```python
from build123d import *

# Parameters (mm, degrees)
BOSS_EXTRUDE2_DEPTH = 5
SKETCH3_W           = 9
SKETCH3_H           = 10
BOSS_EXTRUDE3_DEPTH = 4
SKETCH4_R           = 2.5
CUT_EXTRUDE1_DEPTH  = 10
FILLET1_R           = 1.75


with BuildPart() as part:
    # Sketch1 → Boss-Extrude2 (new body)
    with BuildSketch(Plane(origin=(0, 0, 0), x_dir=(1, 0, 0), z_dir=(0, 1, 0))):
        Polygon((0, 0), (-2, 9), (11, 9), (9, 0), (9, -10), (0, -10), align=None)
    extrude(amount=BOSS_EXTRUDE2_DEPTH)

    # Sketch3 → Boss-Extrude3 (add)
    with BuildSketch(Plane.XZ):
        with Locations((4.5, 5)):
            Rectangle(SKETCH3_W, SKETCH3_H)
    extrude(amount=BOSS_EXTRUDE3_DEPTH)

    # Sketch4 → Cut-Extrude1 (cut, through all)
    with BuildSketch(Plane.XZ.offset(4)):
        with Locations((4.5, 5)):
            Circle(SKETCH4_R)
    extrude(amount=-CUT_EXTRUDE1_DEPTH, mode=Mode.SUBTRACT)

    # Fillet1
    fillet1_edges = [part.edges().sort_by_distance(p)[0] for p in [
        (9, 5, 5),
        (10, 5, -4.5),
        (4.5, 5, -9),
        (-1, 5, -4.5),
        (0, 5, 5),
        (4.5, 5, 10),
    ]]
    fillet(fillet1_edges, radius=FILLET1_R)


solid = part.part
```
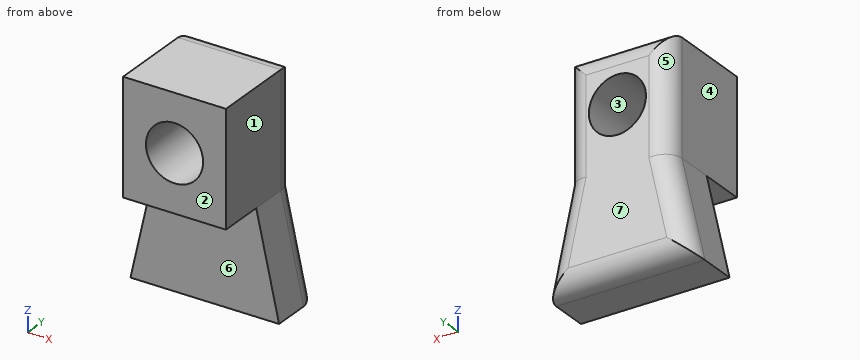
Could you check a few things on this model? Use its own coordinates, in mm. Face numbers are marked on the shaded views. A direction names the side the tool comes from. Coordinates: 2 decimals unless noted, no trailing zeros. Write each loop counter-clockwise with the first axis right and the second up, starting at its lowest first coordinate (ties: lowest second). Pieces come first, ordered by that corner, then holes. Notation, with made-up numbers: (-32, 33) -> (9, 33) arc R18 cw to (9, 39) -> close; hole circle Ø6 at (31, 84). An arc over 180 degrees is marked (long way). One line per question, with ' | ' between items. Start each with the question number.
1. For the marked faces 5, 6 and 7, which set-ups out of +Z, -Z, +X, -X, +Y, -Y let a thin tool reach every point of the face, with its end or its side?
2. Please list where these lines run through material, in increasing order: line 1 along Z through (x, y) = (4.5, -1); line 2 along Y through (x, z) = (6.25, -5.25); line 3 along Z through (x, y) = (4.5, 1.25).
3. If we section it at B-B (x = 4.5): Please give me the cut outline in (y, z), and give its area (3 significant figures).
4. Will these pins go through, and if not, where does the flat tip stop? P1, Ø1.2, axis at x = 3.5, y = -2.5, coming from the -Z side; P2, Ø2, axis at y = 0, z = 2.5, coming from the +X side; P3, Ø3.5, axis at y = 1.5, z = 6, coming from the -X side.
5. If we section it at A-A (z = 3): Please give me the cut outline in (x, y), and give its area (3 significant figures).
6. Thinking about a two-plate mould opening in X: for the marked faces 1, 2, 3 and 4, which applies, pulls with the +X half, pulls with the -X half, needs draft (parallel to the pull), parting line crosses it, or undercut?
7. If we section it at D-D (z = 5): Please give me the cut outline in (x, y), and give its area (3 significant figures).
8. If we section it at C-C (y = 2): Please give me the cut outline in (x, z), and give its area (3 significant figures).
Return value:
1) face 5: +Z, -X, +Y | face 6: -Z, +X, -X, -Y | face 7: +Z, -Z, +X, -X, +Y
2) line 1: z = 0 to 2.5, 7.5 to 10 | line 2: y = 0 to 5 | line 3: z = -9 to 2.5, 7.5 to 10
3) outline: (-4, 0) -> (0, 0) -> (0, -9) -> (3.25, -9) arc R1.75 ccw to (5, -7.25) -> (5, 2.5) -> (-4, 2.5) -> close; (-4, 7.5) -> (5, 7.5) -> (5, 8.25) arc R1.75 ccw to (3.25, 10) -> (-4, 10) -> close | area: 88.7 mm²
4) P1: stops at z = 0 | P2: stops at x = 9 | P3: stops at x = 0
5) outline: (0, -4) -> (3, -4) -> (3, 5) -> (1.75, 5) arc R1.75 ccw to (0, 3.25) -> close; (6, -4) -> (9, -4) -> (9, 3.25) arc R1.75 ccw to (7.25, 5) -> (6, 5) -> close | area: 52.7 mm²
6) face 1: pulls with the +X half | face 2: needs draft | face 3: undercut | face 4: pulls with the -X half
7) outline: (0, -4) -> (2, -4) -> (2, 5) -> (1.75, 5) arc R1.75 ccw to (0, 3.25) -> close; (7, -4) -> (9, -4) -> (9, 3.25) arc R1.75 ccw to (7.25, 5) -> (7, 5) -> close | area: 34.7 mm²
8) outline: (-2, -9) -> (11, -9) -> (9, 0) -> (9, 10) -> (0, 10) -> (0, 0) -> close; hole circle Ø5 at (4.5, 5) | area: 169 mm²
